from build123d import *

# Parameters (mm, degrees)
CYLINDER026_R     = 7
CYLINDER026_DEPTH = 64
BOX019_W          = 24.25
BOX019_H          = 40.85
BOX019_DEPTH      = 4.25
BOX026_W          = 180
BOX026_H          = 4.25
BOX026_DEPTH      = 10.25
BOX017_W          = 200
BOX017_H          = 4.25
BOX017_DEPTH      = 24.25


with BuildPart() as syringe2_cylinder001:
    # Cylinder026 → Cylinder026 (new body)
    with BuildSketch(Plane(origin=(-110, 36.6, 15.125), x_dir=(0, 0, 1), z_dir=(-1, 0, 0))):
        Circle(CYLINDER026_R)
    extrude(amount=CYLINDER026_DEPTH)


with BuildPart() as cube002:
    # Box019 → Box019 (new body)
    with BuildSketch(Plane(origin=(-169.75, 0, 3), x_dir=(0, 0, 1), z_dir=(-1, 0, 0))):
        with Locations((12.125, 20.425)):
            Rectangle(BOX019_W, BOX019_H)
    extrude(amount=BOX019_DEPTH)


with BuildPart() as cube003:
    # Box026 → Box026 (new body)
    with BuildSketch(Plane(origin=(-167, -4.25, 10), x_dir=(1, 0, 0), z_dir=(0, 0, 1))):
        with Locations((90, 2.125)):
            Rectangle(BOX026_W, BOX026_H)
    extrude(amount=BOX026_DEPTH)


with BuildPart() as cut006:
    # Box017 → Box017 (new body)
    with BuildSketch(Plane(origin=(-174, -4.25, 3), x_dir=(1, 0, 0), z_dir=(0, 0, 1))):
        with Locations((100, 2.125)):
            Rectangle(BOX017_W, BOX017_H)
    extrude(amount=BOX017_DEPTH)

    # Cut: cut Cube003
    add(cube003.part, mode=Mode.SUBTRACT)

    # Fusion: union Cube002
    add(cube002.part)

    # Cut006: cut syringe2_cylinder001
    add(syringe2_cylinder001.part, mode=Mode.SUBTRACT)


solid = cut006.part
Build history of the part. All positions in model axes, mm. A direction names the side the tool comes from. Give positions to 0.01 mm unless a question says otherwise; leave off trailing zeros. Order: outer loops, then holes, each group sorted by start corner. A loop starts at its lowest first (then second) coordinate and runs counter-clockwise, first axis right, second up. Notation, with made-up numbers: M 79.5,-31 L 132.5,-31 A23 ccw 132.5,-18 Z; hole C -31,25.5 d8. An arc over 180 degrees is marked long. Put each result on its own line as item: value.
Item 1: Cut at B-B on x = -131. Write the cut outline in (y, z).
Results are:
outline: M -4.25,3 L 0,3 L 0,10 L -4.25,10 Z; M -4.25,20.25 L 0,20.25 L 0,27.25 L -4.25,27.25 Z
Item 2: Which spindle directions (+Z, -Z, +X, -X, +Y, -Y) get a long thin tool onto all of the face, cutting with end or side? Do faces 4 (the face through (-78, -2, 20.25)), 5 (the face through (-174, 19, 15)), 6 (the face through (-73.2, 0, 9.6)). Say none if no direction does.
Results are:
face 4: +Y, -Y
face 5: +Z, -Z, -X, +Y, -Y
face 6: +Z, -Z, +X, +Y
Item 3: Wall check: probe 1 along Z at (x, y) = (-172.75, 36.6) (3 decimals); probe 2 along Z at (x, y) = (-170, 36); probe 3 along X at (y, z) = (21, 9.5). Give the ranges that are in metal, low to high.
Results are:
probe 1: 3 to 8.125, 22.125 to 27.25
probe 2: 3 to 8.15, 22.1 to 27.25
probe 3: -174 to -169.75
Item 4: Cut at A-A on y = 36.6. Write the cut outline in (x, z) (3 decimals), then the cut area to 3 significant figures.
Results are:
outline: M -174,3 L -169.75,3 L -169.75,8.125 L -174,8.125 Z; M -174,22.125 L -169.75,22.125 L -169.75,27.25 L -174,27.25 Z
area: 43.6 mm2
Item 5: Cut at D-D on y = 5.5. Write the cut outline in (x, z), then the cut area to 3 significant figures.
Results are:
outline: M -174,3 L -169.75,3 L -169.75,27.25 L -174,27.25 Z
area: 103 mm2
Item 6: Pull direction Z, two halves, no side cores. Call faces 1 (the face through (-171.845, 29.603, 14.907)), 2 (the face through (-169.75, 16, 15)), 3 (the face through (-95.8, -0.2, 27.25)): +Z half, -Z half, draft (parallel to the pull), parting line (faces both ways), or undercut.
Results are:
face 1: undercut
face 2: draft
face 3: +Z half
Item 7: Cut at C-C on z = 16.75. Write the cut outline in (x, y), then the cut area to 3 significant figures.
Results are:
outline: M -174,-4.25 L -167,-4.25 L -167,0 L -169.75,0 L -169.75,29.79 L -174,29.79 Z; M 13,-4.25 L 26,-4.25 L 26,0 L 13,0 Z
area: 212 mm2
